```python
from build123d import *

# Parameters (mm, degrees)
F0_W     = 200
F0_H     = 200
F1_DEPTH = 3
F3_DEPTH = 3.001
F4_R     = 7.5
F5_DEPTH = 3.001


with BuildPart() as f1:
    # F0 (on Top) → F1 (new body)
    with BuildSketch(Plane.XY):
        Rectangle(F0_W, F0_H)
    extrude(amount=F1_DEPTH)

    # F2 (on face) → F3 (cut, through all)
    with BuildSketch(Plane.XY.offset(3)):
        with BuildLine():
            Line((-75, 100), (-100, 100))
            Line((-100, 100), (-100, 75))
            Line((-100, 75), (-78, 75))
            ThreePointArc((-78, 75), (-72.87868, 72.87868), (-75, 78))
            Line((-75, 78), (-75, 100))
        make_face()
        with BuildLine():
            ThreePointArc((75, 78), (72.87868, 72.87868), (78, 75))
            Line((78, 75), (100, 75))
            Line((100, 75), (100, 100))
            Line((100, 100), (75, 100))
            Line((75, 100), (75, 78))
        make_face()
        with BuildLine():
            Line((-100, -100), (-75, -100))
            Line((-75, -100), (-75, -78))
            ThreePointArc((-75, -78), (-72.87868, -72.87868), (-78, -75))
            Line((-78, -75), (-100, -75))
            Line((-100, -75), (-100, -100))
        make_face()
        with BuildLine():
            Line((100, -75), (78, -75))
            ThreePointArc((78, -75), (72.87868, -72.87868), (75, -78))
            Line((75, -78), (75, -100))
            Line((75, -100), (100, -100))
            Line((100, -100), (100, -75))
        make_face()
    extrude(amount=-F3_DEPTH, mode=Mode.SUBTRACT)

    # F4 (on face) → F5 (cut, through all)
    with BuildSketch(Plane.XY.offset(3)):
        with Locations((-50, 50)):
            Circle(F4_R)
        with Locations((50, 50)):
            Circle(F4_R)
        with Locations((-50, -50)):
            Circle(F4_R)
        with Locations((50, -50)):
            Circle(F4_R)
    extrude(amount=-F5_DEPTH, mode=Mode.SUBTRACT)


solid = f1.part
```
CAD build for the part. Positions are in the model's coordinates, mm. Give positions to 0.01 mm unless a question says otherwise; leave off trailing zeros. Loops run counter-clockwise (first coordinate to the right, second up) from the corner with the lowest first, then second, coordinate; pieces in that order, holes last. Notation, with made-up numbers: (-23, -14.75) - (16, -14.75) arc R18 ccw to (16, 13.25) - close; hole circle Ø10 at (56.25, 25). An arc over 180 degrees is marked (long way). Put each result on its own line as item: value.
Q1. Mould opens along X. For faces 1 (the face through (-1, 1, 0)), 2 (the face through (48.37, 42.68, 1.52)) say: pulls with the +X half, pulls with the -X half, needs draft (parallel to the pull), parting line crosses it, or undercut.
Filled in:
face 1: needs draft
face 2: undercut
Q2. Slice it at A-A (y = -50). Give the cut face in (x, z), plus the area to 3 significant figures.
Filled in:
outline: (-100, 0) - (-57.5, 0) - (-57.5, 3) - (-100, 3) - close; (-42.5, 0) - (42.5, 0) - (42.5, 3) - (-42.5, 3) - close; (57.5, 0) - (100, 0) - (100, 3) - (57.5, 3) - close
area: 510 mm²
Q3. Probe line 1 along Y through (x, z) = (50, 0.7); line 2 along Y through (x, z) = (51, 1.4); line 3 along X through (y, z) = (85, 2.2). List the from-to ranges inside material, lowest first.
Filled in:
line 1: y = -100 to -57.5, -42.5 to 42.5, 57.5 to 100
line 2: y = -100 to -57.43, -42.57 to 42.57, 57.43 to 100
line 3: x = -75 to 75
Q4. Flat gauge pins, fed straight in: pin 1 (10 mm diameter, centred on x = -2, y = -40, fed in from -Z); pin 2 (1.5 mm diameter, centred on y = 88.5, z = 1.5, fed in from +X); pin 3 (3.5 mm diameter, centred on x = -75, y = -75, fed in from +Z); pin 4 (1.5 mm diameter, centred on y = -88.5, z = 1.5, fed in from -X). Where does each tip first touch, or does it go through?
Filled in:
pin 1: stops at z = 0
pin 2: stops at x = 75
pin 3: passes through
pin 4: stops at x = -75
Q5. Slice it at C-C (z = 0.75). Give the cut face in (x, y), plus the area to 3 significant figures.
Filled in:
outline: (-100, -75) - (-78, -75) arc R3 cw (long way) to (-75, -78) - (-75, -100) - (75, -100) - (75, -78) arc R3 cw (long way) to (78, -75) - (100, -75) - (100, 75) - (78, 75) arc R3 cw (long way) to (75, 78) - (75, 100) - (-75, 100) - (-75, 78) arc R3 cw (long way) to (-78, 75) - (-100, 75) - close; hole circle Ø15 at (-50, -50); hole circle Ø15 at (-50, 50); hole circle Ø15 at (50, -50); hole circle Ø15 at (50, 50)
area: 36,700 mm²
